```python
from build123d import *

# Parameters (mm, degrees)
BOX010_W          = 6.2
BOX010_H          = 10
BOX010_DEPTH      = 2.4
BOX011_W          = 6.2
BOX011_H          = 10
BOX011_DEPTH      = 2.4
CYLINDER008_R     = 1.5
CYLINDER008_DEPTH = 20
CYLINDER007_R     = 1.5
CYLINDER007_DEPTH = 20
CYLINDER006_R     = 4.5
CYLINDER006_DEPTH = 120


with BuildPart() as nut1:
    # Box010 → Box010 (new body)
    with BuildSketch(Plane(origin=(-3.1, -5, 6), x_dir=(1, 0, 0), z_dir=(0, 0, 1))):
        with Locations((3.1, 5)):
            Rectangle(BOX010_W, BOX010_H)
    extrude(amount=BOX010_DEPTH)


with BuildPart() as nut2:
    # Box011 → Box011 (new body)
    with BuildSketch(Plane(origin=(-3.1, -5, 111.6), x_dir=(1, 0, 0), z_dir=(0, 0, 1))):
        with Locations((3.1, 5)):
            Rectangle(BOX011_W, BOX011_H)
    extrude(amount=BOX011_DEPTH)


with BuildPart() as columnhole2:
    # Cylinder008 → Cylinder008 (new body)
    with BuildSketch(Plane.XY.offset(100)):
        Circle(CYLINDER008_R)
    extrude(amount=CYLINDER008_DEPTH)


with BuildPart() as columnhole1:
    # Cylinder007 → Cylinder007 (new body)
    with BuildSketch(Plane.XY):
        Circle(CYLINDER007_R)
    extrude(amount=CYLINDER007_DEPTH)


with BuildPart() as column:
    # Cylinder006 → Cylinder006 (new body)
    with BuildSketch(Plane.XY):
        Circle(CYLINDER006_R)
    extrude(amount=CYLINDER006_DEPTH)

    # Cut010: cut ColumnHole1
    add(columnhole1.part, mode=Mode.SUBTRACT)

    # Cut011: cut ColumnHole2
    add(columnhole2.part, mode=Mode.SUBTRACT)

    # Cut012: cut Nut2
    add(nut2.part, mode=Mode.SUBTRACT)

    # Cut013: cut Nut1
    add(nut1.part, mode=Mode.SUBTRACT)


solid = column.part
```
The listing builds one solid part. Answer for the finished solid, in the listing's coordinates (mm). A direction names the side the tool comes from. Give positions to 0.01 mm unless a question says otherwise; leave off trailing zeros. Write each loop counter-clockwise with the first axis right and the second up, starting at its lowest first coordinate (ties: lowest second). Pieces come first, ordered by that corner, then holes. Notation, with made-up numbers: (43.5, 32.25) -> (88.5, 32.25) arc R32 cw to (88.5, 64.25) -> close; hole circle Ø1 at (33, -19.75). An arc over 180 degrees is marked (long way). Use one line per item in the form item = value.
1) Section A-A on x = 0 is taken. Write down the section's boundary in (y, z).
Result:
outline = (-4.5, 0) -> (-1.5, 0) -> (-1.5, 6) -> (-4.5, 6) -> close; (-4.5, 8.4) -> (-1.5, 8.4) -> (-1.5, 20) -> (1.5, 20) -> (1.5, 8.4) -> (4.5, 8.4) -> (4.5, 111.6) -> (1.5, 111.6) -> (1.5, 100) -> (-1.5, 100) -> (-1.5, 111.6) -> (-4.5, 111.6) -> close; (-4.5, 114) -> (-1.5, 114) -> (-1.5, 120) -> (-4.5, 120) -> close; (1.5, 0) -> (4.5, 0) -> (4.5, 6) -> (1.5, 6) -> close; (1.5, 114) -> (4.5, 114) -> (4.5, 120) -> (1.5, 120) -> close
2) Section C-C on z = 108 is taken. Write down the section's boundary in (x, y).
Result:
outline = circle Ø9 at (0, 0); hole circle Ø3 at (0, 0)
3) Straight lines are drawn through the part: probe 1 along Z at (x, y) = (-1.5, 0.5); probe 2 along Y at (x, z) = (0, 13.5); probe 3 along Z at (x, y) = (1, -0.75). For each, find the intervals that lie inside material, in ascending order.
Result:
probe_1 = 0 to 6, 8.4 to 111.6, 114 to 120
probe_2 = -4.5 to -1.5, 1.5 to 4.5
probe_3 = 20 to 100
4) Section B-B on y = 0 is taken. Write down the section's boundary in (x, z).
Result:
outline = (-4.5, 0) -> (-1.5, 0) -> (-1.5, 6) -> (-3.1, 6) -> (-3.1, 8.4) -> (-1.5, 8.4) -> (-1.5, 20) -> (1.5, 20) -> (1.5, 8.4) -> (3.1, 8.4) -> (3.1, 6) -> (1.5, 6) -> (1.5, 0) -> (4.5, 0) -> (4.5, 120) -> (1.5, 120) -> (1.5, 114) -> (3.1, 114) -> (3.1, 111.6) -> (1.5, 111.6) -> (1.5, 100) -> (-1.5, 100) -> (-1.5, 111.6) -> (-3.1, 111.6) -> (-3.1, 114) -> (-1.5, 114) -> (-1.5, 120) -> (-4.5, 120) -> close
5) A tool of negligible diameter and unlimited length cuts with its end or side. For faces 1 (the cylindrical face through (-1.5, 0.07, 116.96)), 2 (the cylindrical face through (-1.5, 0.07, 14.12)), 3 (the flat face through (-1.4, -0.9, 8.4)), from which of +Z, -Z, +X, -X, +Y, -Y can it reach the whole face along a straight path? Write none if from no direction.
Result:
face_1 = +Z
face_2 = -Z
face_3 = +Y, -Y
6) For a pull along X with two mould halves and no side action, classify faces 4 (the flat face through (-1.4, -0.9, 6)), 5 (the flat face through (0, -2, 0)), 6 (the cylindrical face through (-4.496, 0.198, 59.16)) as +X half, -X half, draft (parallel to the pull), parting line (faces both ways), or undercut.
Result:
face_4 = undercut
face_5 = draft
face_6 = parting line
7) Section D-D on z = 81.5 is taken. Write down the section's boundary in (x, y), plus the area to 3 significant figures.
Result:
outline = circle Ø9 at (0, 0)
area = 63.6 mm²
8) Each of these flat-tipped pins is pushed along its axis until it touches: P1, Ø3, axis at y = -2.5, z = 66.5, coming from the -X side; P2, Ø0.9, axis at x = -0.5, y = 0, coming from the -Z side; P3, Ø1.2, axis at y = -1, z = 7.5, coming from the -X side. Where does it stop, or does it pass through?
Result:
P1 = -4.39
P2 = 20
P3 = -4.48
